```python
from build123d import *

# Parameters (mm, degrees)
SKETCH1_R           = 2
SKETCH1_R_2         = 1.6
BOSS_EXTRUDE1_DEPTH = 3.175
FILLET1_R           = 3


with BuildPart() as part:
    # Sketch1 → Boss-Extrude1 (new body)
    with BuildSketch(Plane(origin=(0, 0, 0), x_dir=(1, 0, 0), z_dir=(0, 1, 0))):
        Polygon((-130, -300), (-94, -300), (-94, 200), (94, 200), (94, -300), (130, -300), (130, 300), (-130, 300), align=None)
        with Locations(Location((120, 290, 0), (0, 0, 270))):
            Circle(SKETCH1_R, mode=Mode.SUBTRACT)
        with Locations(Location((120, 232, 0), (0, 0, 270))):
            Circle(SKETCH1_R, mode=Mode.SUBTRACT)
        with Locations(Location((120, 174, 0), (0, 0, 270))):
            Circle(SKETCH1_R, mode=Mode.SUBTRACT)
        with Locations(Location((120, 116, 0), (0, 0, 270))):
            Circle(SKETCH1_R, mode=Mode.SUBTRACT)
        with Locations(Location((120, 58, 0), (0, 0, 270))):
            Circle(SKETCH1_R, mode=Mode.SUBTRACT)
        with Locations(Location((120, 0, 0), (0, 0, 270))):
            Circle(SKETCH1_R, mode=Mode.SUBTRACT)
        with Locations(Location((120, -58, 0), (0, 0, 270))):
            Circle(SKETCH1_R, mode=Mode.SUBTRACT)
        with Locations(Location((120, -116, 0), (0, 0, 270))):
            Circle(SKETCH1_R, mode=Mode.SUBTRACT)
        with Locations(Location((120, -174, 0), (0, 0, 270))):
            Circle(SKETCH1_R, mode=Mode.SUBTRACT)
        with Locations(Location((120, -232, 0), (0, 0, 270))):
            Circle(SKETCH1_R, mode=Mode.SUBTRACT)
        with Locations(Location((120, -290, 0), (0, 0, 270))):
            Circle(SKETCH1_R, mode=Mode.SUBTRACT)
        with Locations(Location((-120, 232, 0), (0, 0, 90))):
            Circle(SKETCH1_R, mode=Mode.SUBTRACT)
        with Locations(Location((-120, -290, 0), (0, 0, 90))):
            Circle(SKETCH1_R, mode=Mode.SUBTRACT)
        with Locations(Location((-120, -232, 0), (0, 0, 90))):
            Circle(SKETCH1_R, mode=Mode.SUBTRACT)
        with Locations(Location((-120, -174, 0), (0, 0, 90))):
            Circle(SKETCH1_R, mode=Mode.SUBTRACT)
        with Locations(Location((-120, -116, 0), (0, 0, 90))):
            Circle(SKETCH1_R, mode=Mode.SUBTRACT)
        with Locations(Location((-120, -58, 0), (0, 0, 90))):
            Circle(SKETCH1_R, mode=Mode.SUBTRACT)
        with Locations(Location((-120, 0, 0), (0, 0, 90))):
            Circle(SKETCH1_R, mode=Mode.SUBTRACT)
        with Locations(Location((-120, 58, 0), (0, 0, 90))):
            Circle(SKETCH1_R, mode=Mode.SUBTRACT)
        with Locations(Location((-120, 116, 0), (0, 0, 90))):
            Circle(SKETCH1_R, mode=Mode.SUBTRACT)
        with Locations(Location((-120, 174, 0), (0, 0, 90))):
            Circle(SKETCH1_R, mode=Mode.SUBTRACT)
        with Locations(Location((-120, 290, 0), (0, 0, 90))):
            Circle(SKETCH1_R, mode=Mode.SUBTRACT)
        with Locations(Location((112, 235, 0), (0, 0, 270))):
            Circle(SKETCH1_R_2, mode=Mode.SUBTRACT)
        with Locations(Location((-112, 235, 0), (0, 0, 90))):
            Circle(SKETCH1_R_2, mode=Mode.SUBTRACT)
        with Locations(Location((112, -235, 0), (0, 0, 90))):
            Circle(SKETCH1_R_2, mode=Mode.SUBTRACT)
        with Locations(Location((-112, -235, 0), (0, 0, 270))):
            Circle(SKETCH1_R_2, mode=Mode.SUBTRACT)
        with Locations(Location((104, 290, 0), (0, 0, 270))):
            Circle(SKETCH1_R, mode=Mode.SUBTRACT)
        with Locations(Location((104, 232, 0), (0, 0, 270))):
            Circle(SKETCH1_R, mode=Mode.SUBTRACT)
        with Locations(Location((104, 174, 0), (0, 0, 270))):
            Circle(SKETCH1_R, mode=Mode.SUBTRACT)
        with Locations(Location((104, 116, 0), (0, 0, 270))):
            Circle(SKETCH1_R, mode=Mode.SUBTRACT)
        with Locations(Location((104, 58, 0), (0, 0, 270))):
            Circle(SKETCH1_R, mode=Mode.SUBTRACT)
        with Locations(Location((104, 0, 0), (0, 0, 270))):
            Circle(SKETCH1_R, mode=Mode.SUBTRACT)
        with Locations(Location((104, -58, 0), (0, 0, 270))):
            Circle(SKETCH1_R, mode=Mode.SUBTRACT)
        with Locations(Location((104, -116, 0), (0, 0, 270))):
            Circle(SKETCH1_R, mode=Mode.SUBTRACT)
        with Locations(Location((104, -174, 0), (0, 0, 270))):
            Circle(SKETCH1_R, mode=Mode.SUBTRACT)
        with Locations(Location((104, -232, 0), (0, 0, 270))):
            Circle(SKETCH1_R, mode=Mode.SUBTRACT)
        with Locations(Location((104, -290, 0), (0, 0, 270))):
            Circle(SKETCH1_R, mode=Mode.SUBTRACT)
        with Locations(Location((-104, -290, 0), (0, 0, 90))):
            Circle(SKETCH1_R, mode=Mode.SUBTRACT)
        with Locations(Location((-104, -232, 0), (0, 0, 90))):
            Circle(SKETCH1_R, mode=Mode.SUBTRACT)
        with Locations(Location((-104, -174, 0), (0, 0, 90))):
            Circle(SKETCH1_R, mode=Mode.SUBTRACT)
        with Locations(Location((-104, -116, 0), (0, 0, 90))):
            Circle(SKETCH1_R, mode=Mode.SUBTRACT)
        with Locations(Location((-104, -58, 0), (0, 0, 90))):
            Circle(SKETCH1_R, mode=Mode.SUBTRACT)
        with Locations(Location((-104, 0, 0), (0, 0, 90))):
            Circle(SKETCH1_R, mode=Mode.SUBTRACT)
        with Locations(Location((-104, 58, 0), (0, 0, 90))):
            Circle(SKETCH1_R, mode=Mode.SUBTRACT)
        with Locations(Location((-104, 116, 0), (0, 0, 90))):
            Circle(SKETCH1_R, mode=Mode.SUBTRACT)
        with Locations(Location((-104, 174, 0), (0, 0, 90))):
            Circle(SKETCH1_R, mode=Mode.SUBTRACT)
        with Locations(Location((-104, 232, 0), (0, 0, 90))):
            Circle(SKETCH1_R, mode=Mode.SUBTRACT)
        with Locations(Location((-104, 290, 0), (0, 0, 90))):
            Circle(SKETCH1_R, mode=Mode.SUBTRACT)
        with Locations(Location((112, 0, 0), (0, 0, 270))):
            Circle(SKETCH1_R_2, mode=Mode.SUBTRACT)
        with Locations(Location((-112, 0, 0), (0, 0, 90))):
            Circle(SKETCH1_R_2, mode=Mode.SUBTRACT)
        with Locations(Location((-72, 290, 0), (0, 0, 90))):
            Circle(SKETCH1_R, mode=Mode.SUBTRACT)
        with Locations(Location((-40, 290, 0), (0, 0, 90))):
            Circle(SKETCH1_R, mode=Mode.SUBTRACT)
        with Locations(Location((-8, 290, 0), (0, 0, 90))):
            Circle(SKETCH1_R, mode=Mode.SUBTRACT)
        with Locations(Location((24, 290, 0), (0, 0, 90))):
            Circle(SKETCH1_R, mode=Mode.SUBTRACT)
        with Locations(Location((56, 290, 0), (0, 0, 90))):
            Circle(SKETCH1_R, mode=Mode.SUBTRACT)
        with Locations(Location((88, 290, 0), (0, 0, 90))):
            Circle(SKETCH1_R, mode=Mode.SUBTRACT)
        with Locations(Location((-72, 232, 0), (0, 0, 90))):
            Circle(SKETCH1_R, mode=Mode.SUBTRACT)
        with Locations(Location((-40, 232, 0), (0, 0, 90))):
            Circle(SKETCH1_R, mode=Mode.SUBTRACT)
        with Locations(Location((-8, 232, 0), (0, 0, 90))):
            Circle(SKETCH1_R, mode=Mode.SUBTRACT)
        with Locations(Location((24, 232, 0), (0, 0, 90))):
            Circle(SKETCH1_R, mode=Mode.SUBTRACT)
        with Locations(Location((56, 232, 0), (0, 0, 90))):
            Circle(SKETCH1_R, mode=Mode.SUBTRACT)
        with Locations(Location((88, 232, 0), (0, 0, 90))):
            Circle(SKETCH1_R, mode=Mode.SUBTRACT)
    extrude(amount=BOSS_EXTRUDE1_DEPTH)

    # Fillet1
    fillet1_edges = [part.edges().sort_by_distance(p)[0] for p in [
        (130, 1.5875, 300),
        (94, 1.5875, 300),
        (94, 1.5875, -200),
        (-94, 1.5875, -200),
        (-94, 1.5875, 300),
        (-130, 1.5875, 300),
        (-130, 1.5875, -300),
        (130, 1.5875, -300),
    ]]
    fillet(fillet1_edges, radius=FILLET1_R)


solid = part.part
```
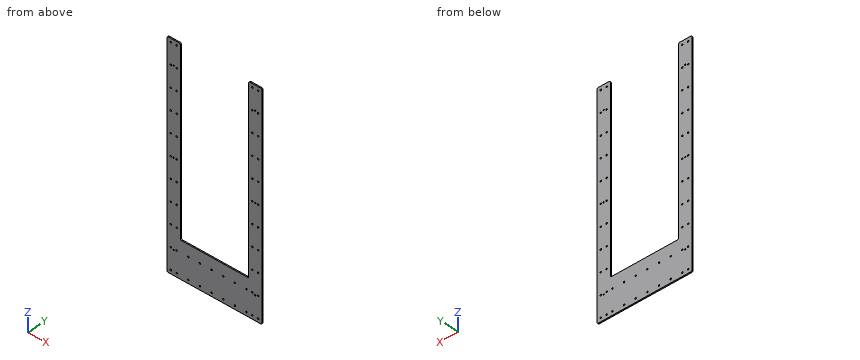
Can you work these out from the model? Positions are in its coordinate system, mm. Coordinates: 2 decimals unless noted, no trailing zeros. Loops run counter-clockwise (first coordinate to the right, second up) from the corner with the lowest first, then second, coordinate; pieces in that order, holes last.
1) Imagine slicing it at C-C on y = 1.35. State how many separate pieces and enclosed holes the cut face has, plus the area to 3 significant figures.
2) Imagine slicing it at A-A on z = 40. List the corners of the cut face in (x, y) for me (3 decimals).
3) I need wall thicknesses on probe 1 along X at (y, z) = (1.25, 290); probe 2 along Z at (x, y) = (112, 0.8); probe 3 along X at (y, z) = (1.95, 104). Which ranges of each line are inside material? Lowest first, please.
4) Imagine slicing it at B-B on x = 64.5. List the corners of the cut face in (y, z) for me (3 decimals), plus the area to 4 significant figures.
Completed:
1. separate pieces: 1
1. enclosed holes: 62
1. area: 61,200 mm2
2. outline: (-130, 0) - (-94, 0) - (-94, 3.175) - (-130, 3.175) - close; (94, 0) - (130, 0) - (130, 3.175) - (94, 3.175) - close
3. probe 1: x = -130 to -122, -118 to -106, -102 to -94, 94 to 102, 106 to 118, 122 to 130
3. probe 2: z = -300 to -236.6, -233.4 to -1.6, 1.6 to 233.4, 236.6 to 300
3. probe 3: x = -130 to -94, 94 to 130
4. outline: (0, -300) - (3.175, -300) - (3.175, -200) - (0, -200) - close
4. area: 317.5 mm2
